Study the drawing (mm; zero at the part's minimum x, y, z) and answer. A direction names the side the tool comes from. Give positions to 0.01 mm unless a question says otherwise; leave off trailing zeros. Loops run counter-clockwise (first coordinate to the right, second up) from the corner with the lowest first, then second, coordinate; pieces in that order, holes last. Notation, with made-up numbers: M -30,33 L 26,33 A20 cw 26,64 Z; hole C 77.5,-6.75 d7. An arc over 180 degrees is marked long. Use one line per item in the form item = value. Start each with the question number.
1. The part is cut by section C-C (x = 75). Write down the section's boundary in (y, z).
2. Straight lines are drawn through the part: line 1 (Z direction, x = 98, y = 14); line 2 (Y direction, x = 105, z = 7.25); line 3 (X direction, y = 23.5, z = 6). For each, find the intervals that lie inside material, in ascending order. Write a range as from..to.
3. Each of these flat-tipped pins is pushed along its axis until it touches: pin 1 Ø10 at (x, y) = (31.5, 36.5) entering from +Z; pin 2 Ø6 at (x, z) = (102, 13.5) entering from +Y; pin 3 Ø4 at (x, z) = (78, 18.5) entering from -Y. Where does it stop, or does it pass through?
4. The part is cut by section A-A (y = 25). Write down the section's boundary in (x, z), and give its area (3 significant figures).
5. For the marked faces 1 and 2, determine the directions among +Z, -Z, +X, -X, +Y, -Y from which every point of the face is accessible in a straight line to the end or side of a thin tool.
6. The part is cut by section B-B (x = 25). Write down the section's boundary in (y, z), and give its area (3 significant figures).
7. The part is cut by section D-D (z = 15.5). Write down the section's boundary in (x, y).
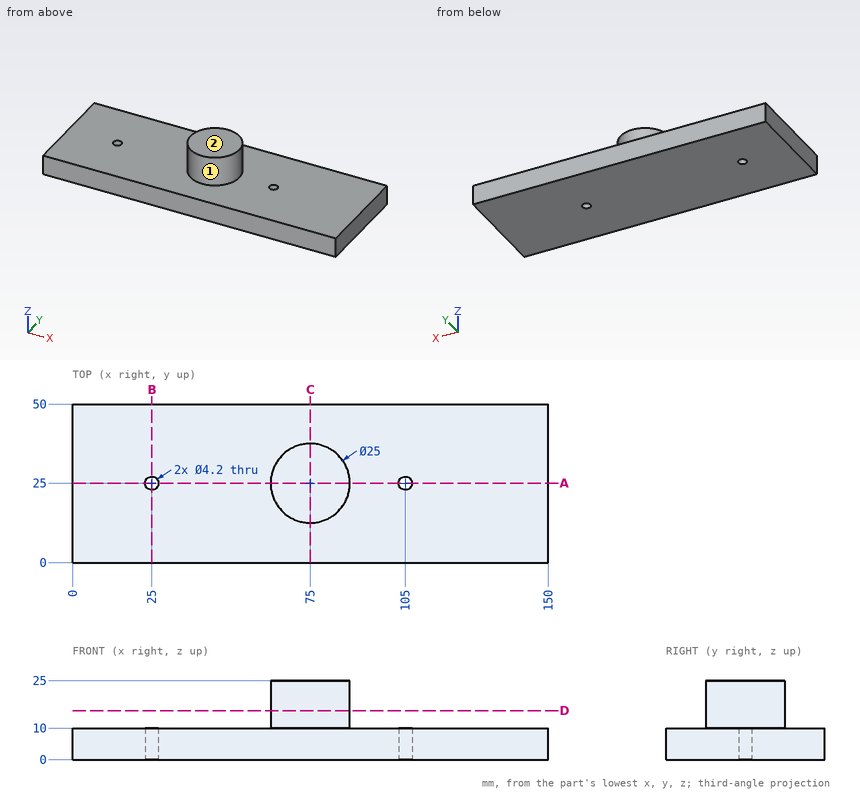
Derived:
q1.outline = M 0,0 L 50,0 L 50,10 L 37.5,10 L 37.5,25 L 12.5,25 L 12.5,10 L 0,10 Z
q2.line_1 = 0..10
q2.line_2 = 0..22.9, 27.1..50
q2.line_3 = 0..23.53, 26.47..103.53, 106.47..150
q3.pin_1 = 10
q3.pin_2 = through
q3.pin_3 = 12.54
q4.outline = M 0,0 L 22.9,0 L 22.9,10 L 0,10 Z; M 27.1,0 L 102.9,0 L 102.9,10 L 87.5,10 L 87.5,25 L 62.5,25 L 62.5,10 L 27.1,10 Z; M 107.1,0 L 150,0 L 150,10 L 107.1,10 Z
q4.area = 1,790 mm2
q5.face_1 = +Z
q5.face_2 = +Z, +X, -X, +Y, -Y
q6.outline = M 0,0 L 22.9,0 L 22.9,10 L 0,10 Z; M 27.1,0 L 50,0 L 50,10 L 27.1,10 Z
q6.area = 458 mm2
q7.outline = C 75,25 d25
